from build123d import *

# Parameters (mm, degrees)
ESBO_O1_W                = 113
ESBO_O1_H                = 115
RESSALTO_EXTRUS_O1_DEPTH = 30
ESBO_O2_W                = 113
ESBO_O2_H                = 115
ESBO_O2_W_2              = 109
ESBO_O2_H_2              = 111
CORTE_EXTRUS_O1_DEPTH    = 2
FILETE1_R                = 10
FILETE2_R                = 12
ESBO_O3_R                = 7.5
CORTE_EXTRUS_O2_DEPTH    = 2
FILETE3_R                = 2


# Some blends are built 0.0001 mm under size
with BuildPart() as part:
    # Esboço1 → Ressalto-extrusão1 (new body)
    with BuildSketch(Plane(origin=(0, 0, 0), x_dir=(1, 0, 0), z_dir=(0, 1, 0))):
        Rectangle(ESBO_O1_W, ESBO_O1_H)
    extrude(amount=RESSALTO_EXTRUS_O1_DEPTH)

    # Esboço2 → Corte-extrusão1 (cut)
    with BuildSketch(Plane(origin=(0, 30, 0), x_dir=(1, 0, 0), z_dir=(0, 1, 0))):
        Rectangle(ESBO_O2_W, ESBO_O2_H)
        Rectangle(ESBO_O2_W_2, ESBO_O2_H_2, mode=Mode.SUBTRACT)
    extrude(amount=-CORTE_EXTRUS_O1_DEPTH, mode=Mode.SUBTRACT)

    # Filete1
    filete1_edges = [part.edges().sort_by_distance(p)[0] for p in [
        (-56.5, 14, -57.5),
        (56.5, 14, -57.5),
        (56.5, 14, 57.5),
        (-56.5, 14, 57.5),
        (54.5, 29, 55.5),
        (-54.5, 29, 55.5),
        (-54.5, 29, -55.5),
        (54.5, 29, -55.5),
    ]]
    fillet(filete1_edges, radius=FILETE1_R)

    # Filete2
    # the kernel refuses this fillet: 12 mm, written as the material it takes off along each edge
    with BuildSketch(Plane(origin=(44.5, 30, 55.5), x_dir=(0, -1, 0), z_dir=(-1, 0, 0)), Plane(origin=(-44.5, 30, -55.5), x_dir=(0, -1, 0), z_dir=(1, 0, 0))) as filete2_piece_1:
        with BuildLine():
            CenterArc((12, -6.633249581), FILETE2_R, 146.442690238, 33.557309762)
            Line((0, -6.633249581), (-0.24, -6.633249581))
            Line((-0.24, -6.633249581), (-0.24, 0))
            Line((-0.24, 0), (0, 0.24))
            ThreePointArc((0, 0.24), (1, 0.24), (1.8, 0.132664992))
            Line((1.8, 0.132664992), (2, 0))
        make_face()
    extrude(amount=89, mode=Mode.SUBTRACT)
    with BuildSketch(Plane(origin=(-54.5, 30, 45.5), x_dir=(0, -1, 0), z_dir=(0, 0, -1)), Plane(origin=(54.5, 30, -45.5), x_dir=(0, -1, 0), z_dir=(0, 0, 1))) as filete2_piece_2:
        with BuildLine():
            CenterArc((12, -6.633249581), FILETE2_R, 146.442690238, 33.557309762)
            Line((0, -6.633249581), (-0.24, -6.633249581))
            Line((-0.24, -6.633249581), (-0.24, 0))
            Line((-0.24, 0), (0, 0.24))
            ThreePointArc((0, 0.24), (1, 0.24), (1.8, 0.132664992))
            Line((1.8, 0.132664992), (2, 0))
        make_face()
    extrude(amount=91, mode=Mode.SUBTRACT)
    with BuildSketch(Plane(origin=(44.5, 30, -45.5), x_dir=(1, 0, 0), z_dir=(0, 0, 1))) as filete2_piece_3:
        with BuildLine():
            CenterArc((3.366750419, -12), FILETE2_R, 56.442690238, 33.557309762)
            Line((3.366750419, 0), (3.366750419, 0.24))
            Line((3.366750419, 0.24), (10, 0.24))
            Line((10, 0.24), (10.24, 0))
            ThreePointArc((10.24, 0), (10.24, -1), (10.132664992, -1.8))
            Line((10.132664992, -1.8), (10, -2))
        make_face()
    revolve(axis=Axis((44.5, 30, -45.5), (0, 1, 0)), revolution_arc=90, mode=Mode.SUBTRACT)
    with BuildSketch(Plane(origin=(44.5, 30, 45.5), x_dir=(0, 0, 1), z_dir=(-1, 0, 0))) as filete2_piece_4:
        with BuildLine():
            CenterArc((3.366750419, -12), FILETE2_R, 56.442690238, 33.557309762)
            Line((3.366750419, 0), (3.366750419, 0.24))
            Line((3.366750419, 0.24), (10, 0.24))
            Line((10, 0.24), (10.24, 0))
            ThreePointArc((10.24, 0), (10.24, -1), (10.132664992, -1.8))
            Line((10.132664992, -1.8), (10, -2))
        make_face()
    revolve(axis=Axis((44.5, 30, 45.5), (0, 1, 0)), revolution_arc=90, mode=Mode.SUBTRACT)
    with BuildSketch(Plane(origin=(-44.5, 30, -45.5), x_dir=(-1, 0, 0), z_dir=(0, 0, 1))) as filete2_piece_5:
        with BuildLine():
            CenterArc((3.366750419, 12), FILETE2_R, 270, 33.557309762)
            Line((3.366750419, 0), (3.366750419, -0.24))
            Line((3.366750419, -0.24), (10, -0.24))
            Line((10, -0.24), (10.24, 0))
            ThreePointArc((10.24, 0), (10.24, 1), (10.132664992, 1.8))
            Line((10.132664992, 1.8), (10, 2))
        make_face()
    revolve(axis=Axis((-44.5, 30, -45.5), (0, -1, 0)), revolution_arc=90, mode=Mode.SUBTRACT)
    with BuildSketch(Plane(origin=(-44.5, 30, 45.5), x_dir=(-1, 0, 0), z_dir=(0, 0, -1))) as filete2_piece_6:
        with BuildLine():
            CenterArc((3.366750419, -12), FILETE2_R, 56.442690238, 33.557309762)
            Line((3.366750419, 0), (3.366750419, 0.24))
            Line((3.366750419, 0.24), (10, 0.24))
            Line((10, 0.24), (10.24, 0))
            ThreePointArc((10.24, 0), (10.24, -1), (10.132664992, -1.8))
            Line((10.132664992, -1.8), (10, -2))
        make_face()
    revolve(axis=Axis((-44.5, 30, 45.5), (0, 1, 0)), revolution_arc=90, mode=Mode.SUBTRACT)

    # Esboço3 → Corte-extrusão2 (cut)
    with BuildSketch(Plane(origin=(0, 30, 0), x_dir=(1, 0, 0), z_dir=(0, 1, 0))):
        with Locations(Location((-32.866750419, 33.866750419, 0), (0, 0, 270))):
            Circle(ESBO_O3_R)
    extrude(amount=-CORTE_EXTRUS_O2_DEPTH, mode=Mode.SUBTRACT)

    # Filete3
    filete3_edges = [part.edges().sort_by_distance(p)[0] for p in [
        (-32.866750419, 28, -41.366750419),
    ]]
    fillet(filete3_edges, radius=FILETE3_R - 0.0001)  # a hair under: the kernel refuses the full size


solid = part.part
Design review of the part built by this model. Coordinates are the model's own, in mm. Give positions to 0.01 mm unless a question says otherwise; leave off trailing zeros. Use CSV: the item, a comma, the result in double quotes. Start each with the question number.
1. Wall thickness on L1, parallel to Z at x = 47, y = 7.25; L2, parallel to Y at x = -39, z = 49; L3, parallel to Y at x = -33.5, z = -33.5: over which ranges is each line inside the solid? List them lowest first.
2. Insertion check: P1, Ø3.5, axis at x = -35.5, z = -34, coming from the +Y side. The pin has a flat end and moves straight along its axis. Give the tip position at first contact, or say it passes through.
3. Draft analysis for pull direction Z (two halves, no side actions). For faces 1 (the flat face through (56.5, 14, 1)), 2 (the flat face through (-33, 28, -34)), 3 (the flat face through (-1, 14, -57.5)), state which applies: released by +Z, released by -Z, zero draft, split by the parting line, or undercut.
Results found:
1,L1,"z = -57.49 to 57.49"
1,L2,"y = 0 to 30"
1,L3,"y = 0 to 28"
2,P1,"stops at y = 28"
3,face 1,"zero draft"
3,face 2,"undercut"
3,face 3,"released by -Z"
